Model file for the job. Use its own axes, mm. Face numbers are marked on the shaded views. A direction names the side the tool comes from. Coordinates: 2 decimals unless noted, no trailing zeros. Order: outer loops, then holes, each group sorted by start corner. A loop starts at its lowest first (then second) coordinate and runs counter-clockwise, first axis right, second up.
from build123d import *

# Parameters (mm, degrees)
BOSS_EXTRUDE1_DEPTH = 9.525


with BuildPart() as part:
    # Sketch1 → Boss-Extrude1 (new, symmetric)
    with BuildSketch(Plane.XY):
        Polygon((0, 63.5), (31.75, 31.75), (44.901280605, 44.901280605), (44.901280605, 0), (63.5, 0), (31.75, -31.75), (44.901280605, -44.901280605), (0, -44.901280605), (0, -63.5), (-31.75, -31.75), (-44.901280605, -44.901280605), (-44.901280605, 0), (-63.5, 0), (-31.75, 31.75), (-44.901280605, 44.901280605), (0, 44.901280605), align=None)
        with BuildLine():
            Line((-4.7625, 23.207583186), (4.7625, 23.207583186))
            Line((4.7625, 23.207583186), (4.7625, 18.445083186))
            ThreePointArc((4.7625, 18.445083186), (0, -19.05), (-4.7625, 18.445083186))
            Line((-4.7625, 18.445083186), (-4.7625, 23.207583186))
        make_face(mode=Mode.SUBTRACT)
    extrude(amount=BOSS_EXTRUDE1_DEPTH, both=True)


solid = part.part
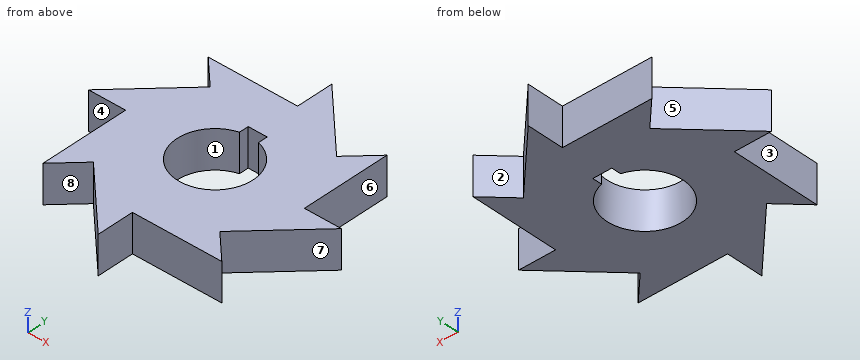
Q1. Which spindle directions (+Z, -Z, +X, -X, +Y, -Y) get a long thin tool onto all of the face, cutting with end or side? Do the marked faces 5, 6, 7 and 8. Say none if no direction does.
Established:
face 5: +Z, -Z, -X
face 6: +Z, -Z, +X, +Y
face 7: +Z, -Z, +X
face 8: +Z, -Z, -Y
Q2. Cut at C-C, the plane y = -24.5. List the corners of the cut face in (x, z) (3 decimals), plus the area to 3 significant figures.
Established:
outline: (-44.901, -9.525) - (39, -9.525) - (39, 9.525) - (-44.901, 9.525) - close
area: 1,600 mm2
Q3. Mould opens along Y. For the marked faces 1, 2, 3 and 4 say: pulls with the +Y half, pulls with the -Y half, needs draft (parallel to the pull), parting line crosses it, or undercut.
Established:
face 1: undercut
face 2: pulls with the +Y half
face 3: needs draft
face 4: pulls with the -Y half
Q4. Probe line 1 (X direction, y = 32, z = -4.75); line 2 (X direction, y = 4, z = 8.75); line 3 (Y direction, x = 7.5, z = 6.5). List the from-to ranges inside material, lowest first.
Established:
line 1: x = -32 to 31.5, 32 to 44.9
line 2: x = -59.5 to -18.63, 18.63 to 44.9
line 3: y = -44.9 to -17.51, 17.51 to 56
Q5. Drop flat-ended pins along their axis: P1, Ø3, axis at x = 15, z = -0.5, coming from the -Y side; P2, Ø9.5, axis at y = -31, z = -2, coming from the -X side; P3, Ø5.5, axis at y = 57.5, z = 3, coming from the -X side. Give the stop position or say it passes through.
Established:
P1: stops at y = -44.9
P2: stops at x = -44.9
P3: stops at x = 0
Q6. Cut at D-D, the plane x = 52. List the corners of the cut face in (y, z) (3 decimals), plus the area to 3 significant figures.
Established:
outline: (-11.5, -9.525) - (0, -9.525) - (0, 9.525) - (-11.5, 9.525) - close
area: 219 mm2
Q7. Cut at A-A, the plane x = 7. List the corners of the cut face in (y, z) (3 decimals), plus the area to 3 significant figures.
Established:
outline: (-44.901, -9.525) - (-17.717, -9.525) - (-17.717, 9.525) - (-44.901, 9.525) - close; (17.717, -9.525) - (56.5, -9.525) - (56.5, 9.525) - (17.717, 9.525) - close
area: 1,260 mm2
Q8. Cut at B-B, the plane z = -2. List the corners of the cut face in (x, y), plus the area to 3 significant figures.
Established:
outline: (-63.5, 0) - (-44.9, 0) - (-44.9, -44.9) - (-31.75, -31.75) - (0, -63.5) - (0, -44.9) - (44.9, -44.9) - (31.75, -31.75) - (63.5, 0) - (44.9, 0) - (44.9, 44.9) - (31.75, 31.75) - (0, 63.5) - (0, 44.9) - (-44.9, 44.9) - (-31.75, 31.75) - close; hole (-4.76, 18.45) arc R19.05 ccw (long way) to (4.76, 18.45) - (4.76, 23.21) - (-4.76, 23.21) - close
area: 6,880 mm2
